Autodesk Inventor part; units mm, degrees
ref_plane "YZ Plane" through (0, 0, 0) normal (1, 0, 0) x (0, 1, 0)
ref_plane "XZ Plane" through (0, 0, 0) normal (0, 1, 0) x (-1, 0, 0)
ref_plane "XY Plane" through (0, 0, 0) normal (0, 0, 1) x (1, 0, 0)
sketch "Sketch1" plane through (0, 0, 0) normal (0, 1, 0) x (-1, 0, 0)
  circle A0 centre (0, 0) radius 35
  circle A1 centre (0, 0) radius 7.5
  dimension "d0" = 70
  dimension "d129" = 15
extrude "Extrusion1" add sketch "Sketch1" along normal blind 4
sketch "Sketch2" plane through (0, 4, 0) normal (0, 1, 0) x (1, 0, 0)
  circle A0 centre (0, 0) radius 30 construction
  point P0 (0, -30)
  point P1 (-25.9808, 15)
  point P2 (25.9808, 15)
  dimension "d130" = 60
  dimension "d131" = 120
  dimension "d132" = 120
hole "Hole1" at (-25.9808, 4, -15) at (25.9808, 4, -15) at (0, 4, 30) direction (0, -1, 0) diameter 3.2 end through all
sketch "Sketch16" plane through (0, 4, 0) normal (0, 1, 0) x (1, 0, 0)
  circle A0 centre (0, 0) radius 12 construction
  point P0 (0, -12)
  point P1 (-10.3923, 6)
  point P2 (10.3923, 6)
  dimension "d155" = 24
  dimension "d156" = 120
  dimension "d157" = 120
hole "Hole14" at (0, 4, 12) at (-10.3923, 4, -6) at (10.3923, 4, -6) direction (0, -1, 0) diameter 2.459 end through all
sketch "Sketch17" plane through (0, 4, 0) normal (0, 1, 0) x (1, 0, 0)
  circle A0 centre (0, 0) radius 12 construction
  point P0 (0, 12)
  point P1 (-10.3923, -6)
  point P2 (10.3923, -6)
  dimension "d165" = 24
  dimension "d166" = 120
  dimension "d167" = 120
hole "Hole15" at (0, 4, -12) at (-10.3923, 4, 6) at (10.3923, 4, 6) direction (0, -1, 0) diameter 3.2 end through all
sketch "Sketch18" plane through (0, 4, 0) normal (0, 1, 0) x (1, 0, 0)
  point P0 (0, 0)
  point P1 (20, 4.5)
  point P2 (20, -4.5)
  dimension "d175" = 9
  dimension "d176" = 4.5
  dimension "d177" = 20
hole "Hole16" at (20, 4, -4.5) at (20, 4, 4.5) direction (0, -1, 0) diameter 2.7 end through all
sketch "Sketch23" plane through (0, 4, 0) normal (0, 1, 0) x (1, 0, 0)
  point P0 (0, 0)
  point P1 (-20, 0)
  dimension "d238" = 20
hole "Hole21" at (-20, 4, 0) direction (0, -1, 0) diameter 4.2 end through all
sketch "Sketch24" plane through (0, 4, 0) normal (0, 1, 0) x (1, 0, 0)
  circle A0 centre (-20, 0) radius 2.1
  point P0 (0, 0)
  point P1 (-20, 6.1)
  point P2 (-20, -6.1)
  dimension "d246" = 12.2
  dimension "d247" = 6.1
hole "Hole22" at (-20, 4, -6.1) at (-20, 4, 6.1) direction (0, -1, 0) diameter 2.013 end through all
pattern_circular "Circular Pattern6" count 3 over 360 about axis through (0, 0, 0) along (0, 1, 0) of "Hole21", "Hole22"
pattern_circular "Circular Pattern7" count 3 over 360 about axis through (0, 0, 0) along (0, 1, 0) of "Hole16"
sketch "Sketch25" plane through (0, 4, 0) normal (0, 1, 0) x (1, 0, 0)
  circle A0 centre (0, 0) radius 30 construction
  circle A1 centre (0, -30) radius 1.6
  point P0 (12.2021, -27.4064)
  point P1 (22.2943, -20.0739)
  point P2 (28.5317, -9.2705)
  point P3 (29.8357, 3.1359)
  dimension "d261" = 60
  dimension "d262" = 24
  dimension "d263" = 24
  dimension "d264" = 24
  dimension "d275" = 24
hole "Hole23" at (22.2943, 4, 20.0739) at (28.5317, 4, 9.2705) at (29.8357, 4, -3.1359) direction (0, -1, 0) diameter 7 end through all
pattern_circular "Circular Pattern8" count 3 over 360 about axis through (0, 0, 0) along (0, 1, 0) of "Hole23"
sketch "Sketch26" plane through (0, 4, 0) normal (0, 1, 0) x (1, 0, 0)
  circle A0 centre (22.2943, -20.0739) radius 3.5
  point P0 (0, 0)
  point P1 (12.2021, -27.4064)
  dimension "d276" = 30
  dimension "d277" = 24
hole "Hole24" at (12.2021, 4, 27.4064) direction (0, -1, 0) diameter 2.459 end through all
pattern_circular "Circular Pattern9" count 3 over 360 about axis through (0, 0, 0) along (0, 1, 0) of "Hole24"
properties part number "torsosc-frame-plate-v3" material "Copper"
CAD build for the part. Positions are in the model's coordinates, mm. Give positions to 0.01 mm unless a question says otherwise; leave off trailing zeros. Write each loop counter-clockwise with the first axis right and the second up, starting at its lowest first coordinate (ties: lowest second). Pieces come first, ordered by that corner, then holes. Notation, with made-up numbers: (24, -17.5) - (30, -17.5) arc R18 ccw to (30, -5.5) - close; hole circle Ø4 at (0, 18). An arc over 180 degrees is marked (long way). Put each result on its own line as item: value.
(1) Saw through at A-A (x = -20). List the corners of the cut face in (y, z).
Working result:
outline: (0, -28.72) - (4, -28.72) - (4, -26.85) - (0, -26.85) - close; (0, -21.69) - (4, -21.69) - (4, -7.11) - (0, -7.11) - close; (0, -5.09) - (4, -5.09) - (4, -2.1) - (0, -2.1) - close; (0, 2.1) - (4, 2.1) - (4, 5.09) - (0, 5.09) - close; (0, 7.11) - (4, 7.11) - (4, 17.43) - (0, 17.43) - close; (0, 22.72) - (4, 22.72) - (4, 28.72) - (0, 28.72) - close
(2) Pull direction Z, two halves, no side cores. Call faces 1 (the flat face through (0, 0, 8)), 2 (the cylindrical face through (-20.954, 1.972, 23.307)), 3 (the cylindrical face through (28, 2, 21)): released by +Z, released by -Z, zero draft, split by the parting line, or undercut.
Working result:
face 1: zero draft
face 2: undercut
face 3: split by the parting line
(3) Saw through at B-B (z = -29). List the corners of the cut face in (x, y), then the cut area to 3 significant figures.
Working result:
outline: (-19.6, 0) - (-9.72, 0) - (-9.72, 4) - (-19.6, 4) - close; (-2.75, 0) - (2.75, 0) - (2.75, 4) - (-2.75, 4) - close; (9.72, 0) - (19.6, 0) - (19.6, 4) - (9.72, 4) - close
area: 101 mm^2
(4) Wall check: L1, parallel to X at y = 2.9, z = -6.1; L2, parallel to Z at x = 30, y = 0.3; L3, parallel to X at y = 1.6, z = -29.5. Give the ranges that are in metal, low to high.
Working result:
L1: -34.46 to -21.01, -18.99 to -11.62, -9.17 to -4.36, 4.36 to 9.17, 11.62 to 27.97, 31.7 to 34.46
L2: -18.03 to -6.63, 0.36 to 6.09, 12.45 to 18.03
L3: -18.83 to -9.73, -2.74 to 2.74, 9.73 to 18.83
(5) Drop flat-ended pins along their axis: pin 1 Ø1 at (y, z) = (1, -21.5) entering from +X; pin 2 Ø1 at (x, y) = (-18.5, 0.5) entering from -Z. Give the stop position or say it passes through.
Working result:
pin 1: x = 28
pin 2: z = -30.02
